Could you check a few things on this model? Use its own coordinates, in mm. Coordinates: 2 decimals unless noted, no trailing zeros. Write each loop counter-clockwise with the first axis right and the second up, starting at its lowest first coordinate (ties: lowest second). Pieces come first, ordered by that corner, then holes. Notation, with made-up numbers: M 86,-17 L 125,-17 A12 cw 125,-3 Z; hole C -11.75,-25.75 d6. An arc over 180 degrees is marked long. Write item = value, one per line.
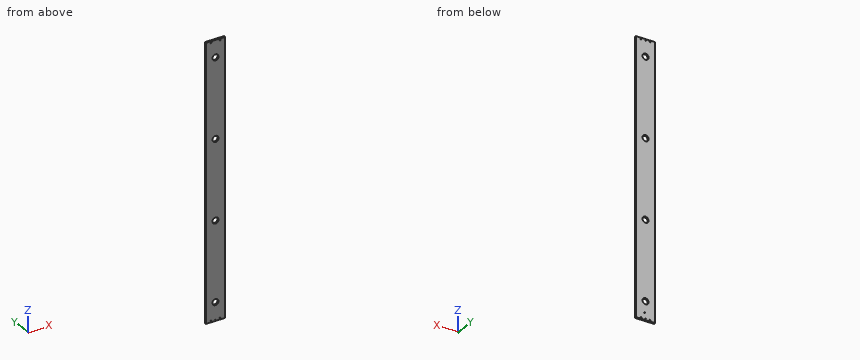
```python
from build123d import *

# Parameters (mm, degrees)
SKETCH1_W                                     = 152.4
SKETCH1_H                                     = 12.7
EXTRUDE_THIN1_DEPTH                           = 1062
CHAMFER1_SIZE                                 = 0.5
CBORE_FOR_1_4_SOCKET_HEAD_CAP_SCREW1_AT_COUNT = 2
CBORE_FOR_1_4_SOCKET_HEAD_CAP_SCREW1_AT_PITCH = 70
EXTRUDE1_REACH                                = 14.7
SKETCH6_R                                     = 23
GUIDE_DIAMETER_DEPTH                          = 13.7
CHAMFER2_SIZE                                 = 0.5
LPATTERN1_COUNT                               = 4
LPATTERN1_PITCH                               = 616
CHAMFER2_OF_LPATTERN1_SIZE                    = 0.5
CHAMFER3_SIZE                                 = 0.5
CUT_EXTRUDE1_DEPTH                            = 2


with BuildPart() as part:
    # Sketch1 → Extrude-Thin1 (new body, symmetric)
    with BuildSketch(Plane.XY):
        Rectangle(SKETCH1_W, SKETCH1_H)
    extrude(amount=EXTRUDE_THIN1_DEPTH, both=True)

    # Chamfer1
    chamfer1_edges = [part.edges().sort_by_distance(p)[0] for p in [
        (0, 6.35, 1062),
        (-76.2, 0, 1062),
        (-76.2, 0, -1062),
        (0, -6.35, 1062),
        (0, 6.35, -1062),
        (76.2, 0, -1062),
        (0, -6.35, -1062),
        (-76.2, -6.35, 0),
        (-76.2, 6.35, 0),
        (76.2, 6.35, 0),
        (76.2, -6.35, 0),
        (76.2, 0, 1062),
    ]]
    chamfer(chamfer1_edges, length=CHAMFER1_SIZE)

    # Sketch3 → CBORE for 1/4 Socket Head Cap Screw1 (revolve, cut)
    with BuildSketch(Plane(origin=(-35, -6.35, -1052), x_dir=(0, 0, -1), z_dir=(1, 0, 0))):
        Polygon((0, 0), (0, 12.7), (4.20624, 12.7), (3.57124, 12.065), (3.57124, 6.35), (5.55625, 6.35), (5.55625, 0), align=None)
    cbore_for_1_4_socket_head_cap_screw1 = revolve(axis=Axis((-35, -12.7, -1052), (0, 1, 0)), mode=Mode.SUBTRACT)

    # CBORE for 1/4 Socket Head Cap Screw1 at: CBORE for 1/4 Socket Head Cap Screw1 ×2
    with Locations(*[(i * CBORE_FOR_1_4_SOCKET_HEAD_CAP_SCREW1_AT_PITCH, 0, 0) for i in range(1, CBORE_FOR_1_4_SOCKET_HEAD_CAP_SCREW1_AT_COUNT)]):
        add(cbore_for_1_4_socket_head_cap_screw1, mode=Mode.SUBTRACT)

    # Sketch4 → 1/8 (0.125) Diameter Hole1 (revolve, cut)
    with BuildSketch(Plane(origin=(0, -6.35, -1052), x_dir=(0, 0, -1), z_dir=(1, 0, 0))):
        Polygon((0, 0), (0, 12.7), (2.2225, 12.7), (1.6002, 12.0777), (1.6002, 0.6223), (2.2225, 0), align=None)
    revolve(axis=Axis((0, -12.7, -1052), (0, 1, 0)), mode=Mode.SUBTRACT)

    # Mirror1: CBORE for 1/4 Socket Head Cap Screw1 across plane
    add(cbore_for_1_4_socket_head_cap_screw1.mirror(Plane.XY), mode=Mode.SUBTRACT)

    # Mirror1 copy 1 sketch → Mirror1 copy 1 (revolve, cut)
    with BuildSketch(Plane(origin=(35, -6.35, 1052), x_dir=(0, 0, 1), z_dir=(1, 0, 0))):
        Polygon((0, 0), (0, -12.7), (4.20624, -12.7), (3.57124, -12.065), (3.57124, -6.35), (5.55625, -6.35), (5.55625, 0), align=None)
    revolve(axis=Axis((35, -12.7, 1052), (0, -1, 0)), mode=Mode.SUBTRACT)

    # Sketch5 → Extrude1 (cut, up to next)
    with BuildSketch(Plane(origin=(0, 6.35, 0), x_dir=(1, 0, 0), z_dir=(0, 1, 0)), mode=Mode.PRIVATE) as extrude1_sk1:
        with BuildLine():
            Line((-1.6002, -1053.5), (-1.6002, -1050.5))
            ThreePointArc((-1.6002, -1050.5), (0, -1048.8998), (1.6002, -1050.5))
            Line((1.6002, -1050.5), (1.6002, -1053.5))
            ThreePointArc((1.6002, -1053.5), (0, -1055.1002), (-1.6002, -1053.5))
        make_face()
    extrude1_tool1 = extrude(extrude1_sk1.sketch, amount=-EXTRUDE1_REACH, mode=Mode.PRIVATE) & part.part
    add(extrude1_tool1.solids().sort_by_distance((0, 6.35, 1052))[0], mode=Mode.SUBTRACT)

    # Sketch6 → guide diameter (cut, through all)
    with BuildSketch(Plane(origin=(0, 6.35, 0), x_dir=(1, 0, 0), z_dir=(0, 1, 0))):
        with Locations(Location((0, 919, 0), (0, 0, 180))):  # turned: the seam where the file's is
            Circle(SKETCH6_R)
    guide_diameter = extrude(amount=-GUIDE_DIAMETER_DEPTH, mode=Mode.SUBTRACT)

    # Chamfer2
    chamfer2_edges = [part.edges().sort_by_distance(p)[0] for p in [
        (23, -6.35, -919),
        (23, 6.35, -919),
    ]]
    chamfer(chamfer2_edges, length=CHAMFER2_SIZE)

    # LPattern1: guide diameter ×4
    with Locations(*[(0, 0, i * LPATTERN1_PITCH) for i in range(1, LPATTERN1_COUNT)]):
        add(guide_diameter, mode=Mode.SUBTRACT)

    # Chamfer2 of LPattern1
    chamfer2_of_lpattern1_edges = [part.edges().sort_by_distance(p)[0] for p in [
        (23, -6.35, -303),
        (23, 6.35, -303),
        (23, -6.35, 313),
        (23, 6.35, 313),
        (23, -6.35, 929),
        (23, 6.35, 929),
    ]]
    chamfer(chamfer2_of_lpattern1_edges, length=CHAMFER2_OF_LPATTERN1_SIZE)

    # Chamfer3
    chamfer3_edges = [part.edges().sort_by_distance(p)[0] for p in [
        (0, 6.35, 1055.1002),
        (1.6002, 6.35, 1052),
        (0, 6.35, 1048.8998),
        (-1.6002, 6.35, 1052),
    ]]
    chamfer(chamfer3_edges, length=CHAMFER3_SIZE)

    # Sketch7 → Cut-Extrude1 (cut)
    with BuildSketch(Plane(origin=(0, 6.35, 0), x_dir=(1, 0, 0), z_dir=(0, 1, 0))):
        with BuildLine():
            Line((10.016442871, 1002.864811478), (10.016442871, 1008.301621094))
            Line((10.016442871, 1008.301621094), (7.08855957, 1008.301621094))
            Line((7.08855957, 1008.301621094), (7.08855957, 1003.295807457))
            add(Edge.make_bspline(
                [(7.08855957, 1003.295807457), (7.085272029, 1003.208940575), (7.079101125, 1003.045886399), (7.035451852, 1002.817641442), (6.955335746, 1002.62460988), (6.843536393, 1002.467570614), (6.70448491, 1002.346963747), (6.545966626, 1002.258305794), (6.364548529, 1002.206474612), (6.237339762, 1002.200801414), (6.17118824, 1002.197851219)],
                knots=[0, 0, 0, 0, 1.285293232, 2.412569968, 3.418386025, 4.354403319, 5.23810445, 6.120527863, 7.022630715, 8, 8, 8, 8], degree=3))
            add(Edge.make_bspline(
                [(6.17118824, 1002.197851219), (6.104964912, 1002.200656064), (5.977618061, 1002.206049755), (5.797214668, 1002.25982572), (5.634101786, 1002.34183535), (5.491945229, 1002.462060899), (5.377499487, 1002.6195556), (5.294517407, 1002.813274474), (5.248231883, 1003.043251768), (5.242447251, 1003.20811075), (5.239370117, 1003.295807457)],
                knots=[0, 0, 0, 0, 0.970712631, 1.866671451, 2.742370236, 3.637940775, 4.57451605, 5.578136324, 6.711690039, 8, 8, 8, 8], degree=3))
            Line((5.239370117, 1003.295807457), (5.239370117, 1008.301621094))
            Line((5.239370117, 1008.301621094), (1.849189453, 1008.301621094))
            Line((1.849189453, 1008.301621094), (1.849189453, 1002.677003174))
            add(Edge.make_bspline(
                [(1.849189453, 1002.677003174), (1.845843655, 1002.587755059), (1.839553911, 1002.419978146), (1.796273178, 1002.183378763), (1.713671661, 1001.983271463), (1.602044928, 1001.817186066), (1.461094123, 1001.68999124), (1.299501043, 1001.595310324), (1.113983026, 1001.54232453), (0.984306529, 1001.534783446), (0.91737133, 1001.530890961)],
                knots=[0, 0, 0, 0, 1.282115211, 2.410239491, 3.433544999, 4.370413449, 5.259840111, 6.137762651, 7.038767785, 8, 8, 8, 8], degree=3))
            add(Edge.make_bspline(
                [(0.91737133, 1001.530890961), (0.851993137, 1001.534651561), (0.726142864, 1001.541890558), (0.545865721, 1001.596390772), (0.387681571, 1001.690646995), (0.247310665, 1001.817205123), (0.134833927, 1001.98271475), (0.056769985, 1002.184311918), (0.008482543, 1002.419532279), (0.002943607, 1002.587655764), (0, 1002.677003174)],
                knots=[0, 0, 0, 0, 0.94634305, 1.821670557, 2.697075277, 3.594139625, 4.539053153, 5.56674892, 6.706875008, 8, 8, 8, 8], degree=3))
            Line((0, 1002.677003174), (0, 1009.197322235))
            add(Edge.make_bspline(
                [(0, 1009.197322235), (0.003403349, 1009.314873529), (0.009736608, 1009.53362358), (0.074602909, 1009.836521786), (0.180649823, 1010.088999186), (0.339573158, 1010.291217597), (0.552801999, 1010.438170066), (0.813387914, 1010.544806157), (1.127716106, 1010.601254331), (1.352976872, 1010.608974714), (1.473572845, 1010.61310791)],
                knots=[0, 0, 0, 0, 1.189944925, 2.214356848, 3.121275872, 3.943259729, 4.783004917, 5.7166381, 6.777575619, 8, 8, 8, 8], degree=3))
            Line((1.473572845, 1010.61310791), (10.392059479, 1010.61310791))
            add(Edge.make_bspline(
                [(10.392059479, 1010.61310791), (10.474780749, 1010.611163402), (10.631859192, 1010.607470999), (10.856621451, 1010.582501559), (11.056627192, 1010.533966149), (11.235432954, 1010.469602563), (11.391264364, 1010.385371213), (11.525717721, 1010.279949262), (11.633961183, 1010.150122691), (11.722671877, 1010.000765575), (11.785939946, 1009.828912547), (11.835213509, 1009.637980919), (11.859793233, 1009.424283611), (11.863628174, 1009.275222133), (11.865632324, 1009.197322235)],
                knots=[0, 0, 0, 0, 1.25760687, 2.388054849, 3.429687073, 4.379296607, 5.269270079, 6.111463577, 6.959732887, 7.823909447, 8.739278143, 9.733531743, 10.815538057, 12, 12, 12, 12], degree=3))
            Line((11.865632324, 1009.197322235), (11.865632324, 1002.864811478))
            add(Edge.make_bspline(
                [(11.865632324, 1002.864811478), (11.862265523, 1002.774764089), (11.855933206, 1002.605401979), (11.812996161, 1002.367164125), (11.730730959, 1002.166636583), (11.618324043, 1002.00251409), (11.478831829, 1001.878582005), (11.319068401, 1001.788356803), (11.138688717, 1001.73440727), (11.01123092, 1001.728799229), (10.945853195, 1001.725922661)],
                knots=[0, 0, 0, 0, 1.303543407, 2.451718649, 3.482873774, 4.417375591, 5.305837532, 6.158811619, 7.05558772, 8, 8, 8, 8], degree=3))
            add(Edge.make_bspline(
                [(10.945853195, 1001.725922661), (10.878836329, 1001.728683151), (10.748933743, 1001.734033965), (10.565169593, 1001.78908629), (10.401495053, 1001.876989185), (10.26161213, 1002.002763084), (10.148391264, 1002.166047339), (10.069867284, 1002.367823404), (10.025886735, 1002.605293266), (10.019721068, 1002.774726352), (10.016442871, 1002.864811478)],
                knots=[0, 0, 0, 0, 0.961524532, 1.863777426, 2.731626687, 3.61454628, 4.543218546, 5.563575511, 6.704588277, 8, 8, 8, 8], degree=3))
        make_face()
    extrude(amount=-CUT_EXTRUDE1_DEPTH, mode=Mode.SUBTRACT)


solid = part.part
```
Item 1: Imagine slicing it at A-A (y = -2). State how many separate pieces and enclosed holes the cut face has, and give its area (3 significant figures).
Numbers:
separate_pieces = 1
enclosed_holes = 10
area = 317,000 mm²
Item 2: Imagine slicing it at B-B (z = 313). Write out the boundary of the cut face in (x, y), and give its area (3 significant figures).
Numbers:
outline = M -76.2,-5.85 L -75.7,-6.35 L -23.5,-6.35 L -23,-5.85 L -23,5.85 L -23.5,6.35 L -75.7,6.35 L -76.2,5.85 Z; M 23,-5.85 L 23.5,-6.35 L 75.7,-6.35 L 76.2,-5.85 L 76.2,5.85 L 75.7,6.35 L 23.5,6.35 L 23,5.85 Z
area = 1,350 mm²
Item 3: If I drill on line 1 along Z through (x, y) = (-35, -2.75); line 2 along X through (y, z) = (4.5, -1052); line 3 along X through (y, z) = (-0.25, -1052), over which ranges is the centre line in solid material (lowest first)?
Numbers:
line_1 = -1062 to -1057.56, -1046.44 to 1046.44, 1057.56 to 1062
line_2 = -76.2 to -38.57, -31.43 to -1.6, 1.6 to 31.43, 38.57 to 76.2
line_3 = -76.2 to -40.56, -29.44 to -1.6, 1.6 to 29.44, 40.56 to 76.2
Item 4: I'm going to push flat-ended pins straight in: P1, Ø6.5, axis at x = 35, z = -1052, coming from the -Y side; P2, Ø9, axis at x = -35, z = 1052, coming from the -Y side. Where does each tip first touch, or does it pass through?
Numbers:
P1 = through
P2 = 0
